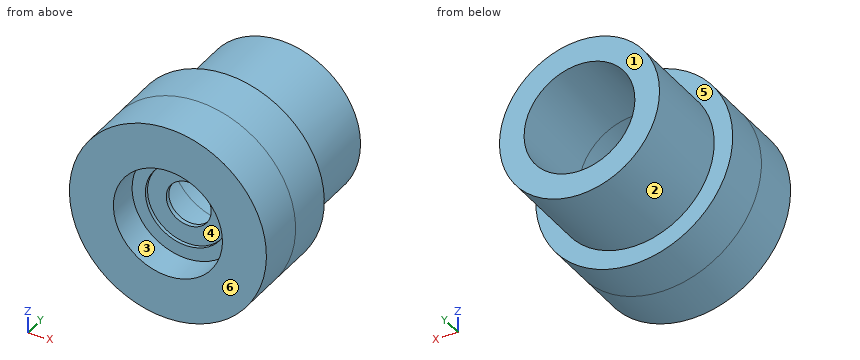
```python
from build123d import *

# Parameters (mm, degrees)
SKETCH1_R           = 20.32
SKETCH1_R_2         = 4.6355
BOSS_EXTRUDE1_DEPTH = 10
SKETCH2_R           = 16.51
SKETCH2_R_2         = 11.43
BOSS_EXTRUDE2_DEPTH = 19.05
BOSS_EXTRUDE3_START = 10.16
SKETCH3_R           = 20.32
SKETCH3_R_2         = 4.6355
BOSS_EXTRUDE3_DEPTH = 10.16
CUT_EXTRUDE1_START  = -12
SKETCH4_R           = 11.43
CUT_EXTRUDE1_DEPTH  = 12
SKETCH6_R           = 11.25
CUT_EXTRUDE3_DEPTH  = 6.5
SKETCH7_R           = 8.5
CUT_EXTRUDE4_DEPTH  = 0.75


with BuildPart() as part:
    # Sketch1 → Boss-Extrude1 (new body)
    with BuildSketch(Plane(origin=(0, 0, 0), x_dir=(1, 0, 0), z_dir=(0, 1, 0))):
        with Locations(Location((0, 0, 0), (0, 0, 270))):
            Circle(SKETCH1_R)
        with Locations(Location((0, 0, 0), (0, 0, 270))):
            Circle(SKETCH1_R_2, mode=Mode.SUBTRACT)
    extrude(amount=BOSS_EXTRUDE1_DEPTH)

    # Sketch2 → Boss-Extrude2 (add)
    with BuildSketch(Plane(origin=(0, 10, 0), x_dir=(1, 0, 0), z_dir=(0, 1, 0))):
        with Locations(Location((0, 0, 0), (0, 0, 90))):
            Circle(SKETCH2_R)
        with Locations(Location((0, 0, 0), (0, 0, 90))):
            Circle(SKETCH2_R_2, mode=Mode.SUBTRACT)
    extrude(amount=BOSS_EXTRUDE2_DEPTH)

    # Sketch3 → Boss-Extrude3 (add)
    with BuildSketch(Plane(origin=(0, 0, 0), x_dir=(-1, 0, 0), z_dir=(0, -1, 0)).offset(BOSS_EXTRUDE3_START)):
        with Locations(Location((0, 0, 0), (0, 0, 90))):
            Circle(SKETCH3_R)
        with Locations(Location((0, 0, 0), (0, 0, 90))):
            Circle(SKETCH3_R_2, mode=Mode.SUBTRACT)
    extrude(amount=-BOSS_EXTRUDE3_DEPTH)

    # Sketch4 → Cut-Extrude1 (cut)
    with BuildSketch(Plane(origin=(0, 10, 0), x_dir=(1, 0, 0), z_dir=(0, 1, 0)).offset(CUT_EXTRUDE1_START)):
        with Locations(Location((0, 0, 0), (0, 0, 90))):
            Circle(SKETCH4_R)
    extrude(amount=CUT_EXTRUDE1_DEPTH, mode=Mode.SUBTRACT)

    # Sketch6 → Cut-Extrude3 (cut)
    with BuildSketch(Plane.XZ.offset(10.16)):
        with Locations(Location((0, 0, 0), (0, 0, 270))):
            Circle(SKETCH6_R)
    extrude(amount=-CUT_EXTRUDE3_DEPTH, mode=Mode.SUBTRACT)

    # Sketch7 → Cut-Extrude4 (cut)
    with BuildSketch(Plane(origin=(0, -3.66, 0), x_dir=(-1, 0, 0), z_dir=(0, -1, 0))):
        with Locations(Location((0, 0, 0), (0, 0, 90))):
            Circle(SKETCH7_R)
    extrude(amount=-CUT_EXTRUDE4_DEPTH, mode=Mode.SUBTRACT)


solid = part.part
```
Work out the finished part from the listing and answer in its coordinate system (mm). Face numbers are marked on the shaded views. A direction names the side the tool comes from. Give positions to 0.01 mm unless a question says otherwise; leave off trailing zeros. Write each loop counter-clockwise with the first axis right and the second up, starting at its lowest first coordinate (ties: lowest second). Pieces come first, ordered by that corner, then holes.
(1) The part is cut by section D-D on x = 15. Write down the section's boundary in (y, z), plus the area to 3 significant figures.
Final values:
outline: (-10.16, -13.71) - (10, -13.71) - (10, -6.9) - (29.05, -6.9) - (29.05, 6.9) - (10, 6.9) - (10, 13.71) - (-10.16, 13.71) - close
area: 816 mm2
(2) The part is cut by section C-C on y = 26. Write down the section's boundary in (x, z).
Final values:
outline: circle Ø33.02 at (0, 0); hole circle Ø22.86 at (0, 0)
(3) The mould has two halves that part along X. Classify the marked faces 1, 2, 3 and 4: pulls with the +X half, pulls with the -X half, needs draft (parallel to the pull), parting line crosses it, or undercut.
Final values:
face 1: needs draft
face 2: parting line crosses it
face 3: undercut
face 4: undercut
(4) Which of the six approach directions +Z, -Z, +X, -X, +Y, -Y give full straight-line access (tool end or side, diameter ignored) to the marked faces 5 and 6?
Final values:
face 5: +Y
face 6: +Z, -Z, +X, -X, -Y
(5) Straight lines are drawn through the part: line 1 (X direction, y = 6, z = 0); line 2 (X direction, y = -6, z = 0); line 3 (Y direction, x = 17.5, z = 8.5). For each, find the intervals that lie inside material, in ascending order.
Final values:
line 1: x = -20.32 to -11.43, 11.43 to 20.32
line 2: x = -20.32 to -11.25, 11.25 to 20.32
line 3: y = -10.16 to 10
(6) Flat-ended cylindrical pins translate along their axes: pin 1 Ø19.5 at (x, z) = (0, 0) entering from -Y; pin 2 Ø12 at (y, z) = (-3, -10.5) entering from -X; pin 3 Ø5 at (x, z) = (-4, 3) entering from -Y. Find the tip coordinate at first contact, or state that the pin passes through.
Final values:
pin 1: stops at y = -3.66
pin 2: stops at x = -19.82
pin 3: stops at y = -2.91
(7) The part is cut by section A-A on z = 0. Write down the section's boundary in (x, y).
Final values:
outline: (-20.32, -10.16) - (-11.25, -10.16) - (-11.25, -3.66) - (-8.5, -3.66) - (-8.5, -2.91) - (-4.64, -2.91) - (-4.64, -2) - (-11.43, -2) - (-11.43, 29.05) - (-16.51, 29.05) - (-16.51, 10) - (-20.32, 10) - close; (4.64, -2.91) - (8.5, -2.91) - (8.5, -3.66) - (11.25, -3.66) - (11.25, -10.16) - (20.32, -10.16) - (20.32, 10) - (16.51, 10) - (16.51, 29.05) - (11.43, 29.05) - (11.43, -2) - (4.64, -2) - close
(8) The part is cut by section B-B on x = 0. Write down the section's boundary in (y, z), plus the area to 3 significant figures.
Final values:
outline: (-10.16, -20.32) - (10, -20.32) - (10, -16.51) - (29.05, -16.51) - (29.05, -11.43) - (-2, -11.43) - (-2, -4.64) - (-2.91, -4.64) - (-2.91, -8.5) - (-3.66, -8.5) - (-3.66, -11.25) - (-10.16, -11.25) - close; (-10.16, 11.25) - (-3.66, 11.25) - (-3.66, 8.5) - (-2.91, 8.5) - (-2.91, 4.64) - (-2, 4.64) - (-2, 11.43) - (29.05, 11.43) - (29.05, 16.51) - (10, 16.51) - (10, 20.32) - (-10.16, 20.32) - close
area: 571 mm2
